from build123d import *

# Parameters (mm, degrees)
SKETCH4_R          = 3.2385
SKETCH4_R_2        = 2.0955
CUT_EXTRUDE1_DEPTH = 13.7


with BuildPart() as part:
    # Sketch3 → Revolve1 (revolve)
    with BuildSketch(Plane.XY):
        Polygon((30.48, -1.361443582), (50.8, -1.361443582), (50.8, 0.543556418), (48.26, 0.543556418), (48.26, 9.433556418), (50.8, 9.433556418), (50.8, 11.338556418), (30.48, 11.338556418), align=None)
    revolve(axis=Axis((30.48, 11.338556418, 0), (0, -1, 0)))

    # Sketch4 → Cut-Extrude1 (cut, through all)
    with BuildSketch(Plane(origin=(0, 11.338556418, 0), x_dir=(1, 0, 0), z_dir=(0, 1, 0))):
        with Locations((30.48, -10.16)):
            Circle(SKETCH4_R)
        with Locations((22.48, -2.16)):
            Circle(SKETCH4_R_2)
        with Locations((38.48, -2.16)):
            Circle(SKETCH4_R_2)
    extrude(amount=-CUT_EXTRUDE1_DEPTH, mode=Mode.SUBTRACT)


solid = part.part
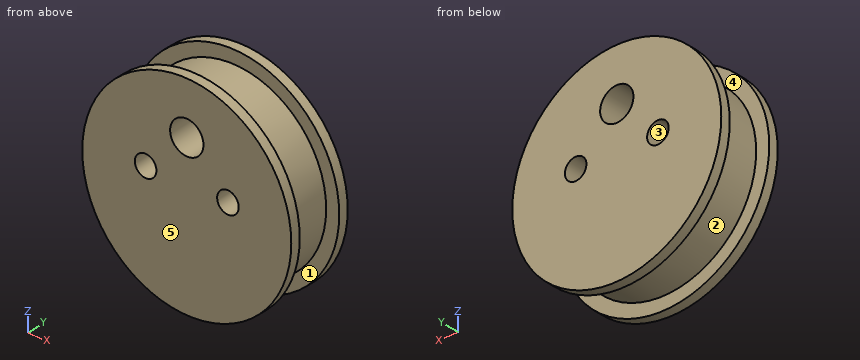
Build history of the part. All positions in model axes, mm. Face numbers are marked on the shaded views. A direction names the side the tool comes from. Round coordinates to 2 decimals unless told otherwise and drop trailing zeros. Write each loop counter-clockwise with the first axis right and the second up, starting at its lowest first coordinate (ties: lowest second). Pieces come first, ordered by that corner, then holes. Notation, with made-up numbers: (40.25, 0.5) - (66.25, 0.5) arc R19 cw to (66.25, 12.5) - close; hole circle Ø7 at (86.5, 54). An arc over 180 degrees is marked (long way). One line per question, with ' | ' between items.
1. Band-saw the part on B-B, the plane y = 8.75. Write the cut outline in (x, z).
Results are:
outline: circle Ø35.56 at (30.48, 0); hole circle Ø4.19 at (22.48, 2.16); hole circle Ø6.48 at (30.48, 10.16); hole circle Ø4.19 at (38.48, 2.16)
2. Band-saw the part on D-D, the plane z = 2.16. Write the cut outline in (x, y), and give its area (3 significant figures).
Results are:
outline: (10.28, -1.36) - (20.38, -1.36) - (20.38, 11.34) - (10.28, 11.34) - (10.28, 9.43) - (12.83, 9.43) - (12.83, 0.54) - (10.28, 0.54) - close; (24.58, -1.36) - (36.38, -1.36) - (36.38, 11.34) - (24.58, 11.34) - close; (40.58, -1.36) - (50.68, -1.36) - (50.68, 0.54) - (48.13, 0.54) - (48.13, 9.43) - (50.68, 9.43) - (50.68, 11.34) - (40.58, 11.34) - close | area: 361 mm^2
3. Band-saw the part on A-A, the plane x = 30.48. Write the cut outline in (y, z), and give its area (3 significant figures).
Results are:
outline: (-1.36, -20.32) - (0.54, -20.32) - (0.54, -17.78) - (9.43, -17.78) - (9.43, -20.32) - (11.34, -20.32) - (11.34, 6.92) - (-1.36, 6.92) - close; (-1.36, 13.4) - (11.34, 13.4) - (11.34, 20.32) - (9.43, 20.32) - (9.43, 17.78) - (0.54, 17.78) - (0.54, 20.32) - (-1.36, 20.32) - close | area: 389 mm^2
4. Tool access for the marked faces 4 and 5: list every direction of +Z, -Z, +X, -X, +Y, -Y with a clear straight run to the whole face (end or side of a thin tool).
Results are:
face 4: none | face 5: +Z, -Z, +X, -X, -Y
5. Mould opens along Z. For the marked faces 1, 2 and 3 say: released by +Z, released by -Z, zero draft, split by the parting line, or undercut.
Results are:
face 1: zero draft | face 2: split by the parting line | face 3: undercut
6. Band-saw the part on C-C, the plane z = 10.16. Write the cut outline in (x, y).
Results are:
outline: (12.88, -1.36) - (27.24, -1.36) - (27.24, 11.34) - (12.88, 11.34) - (12.88, 9.43) - (15.89, 9.43) - (15.89, 0.54) - (12.88, 0.54) - close; (33.72, -1.36) - (48.08, -1.36) - (48.08, 0.54) - (45.07, 0.54) - (45.07, 9.43) - (48.08, 9.43) - (48.08, 11.34) - (33.72, 11.34) - close
7. Drop flat-ended pins along their axis: pin 1 Ø3 at (y, z) = (8.5, 5.5) entering from +X; pin 2 Ø3 at (y, z) = (3, 1) entering from +X; pin 3 Ø5 at (y, z) = (4, -5) entering from -X. Give the stop position or say it passes through.
Results are:
pin 1: x = 50.33 | pin 2: x = 48.26 | pin 3: x = 12.88
8. Drill centre lines: line 1 along Y through (x, z) = (15, -10); line 2 along X through (y, z) = (4, 2.16); line 3 along Z through (x, y) = (38.48, 1). Where is each one in solid material? Low to high. Write a range as from..to.
Results are:
line 1: -1.36..0.54, 9.43..11.34 | line 2: 12.83..20.38, 24.58..36.38, 40.58..48.13 | line 3: -15.88..0.06, 4.26..15.88
